Autodesk Inventor part; units mm, degrees
ref_plane "YZ Plane" through (0, 0, 0) normal (1, 0, 0) x (0, 1, 0)
ref_plane "XZ Plane" through (0, 0, 0) normal (0, 1, 0) x (-1, 0, 0)
ref_plane "XY Plane" through (0, 0, 0) normal (0, 0, 1) x (1, 0, 0)
sketch "Sketch1" plane through (0, 0, 0) normal (0, 0, 1) x (1, 0, 0)
  circle A0 centre (0, 0) radius 6.35
  dimension "d0" = 12.7
extrude "Extrusion1" add sketch "Sketch1" along normal blind 9.652
sketch "Sketch2" plane through (0, 0, 0) normal (0, 0, -1) x (-1, 0, 0)
  circle A0 centre (0, 0) radius 3.302
  dimension "d3" = 6.604
extrude "Extrusion2" add sketch "Sketch2" along normal blind 3.048
chamfer "Chamfer1" distance 0.762 angle 45 1 edges at (-6.35, 0, 9.652) measured on face at (-1.8127, -0.4771, 9.652)
sketch "Sketch3" plane through (0, 0, 9.652) normal (0, 0, 1) x (1, 0, 0)
  circle A0 centre (0, 0) radius 6.35
  line L0 (3.175, 5.4993) -> (6.35, 0)
  line L1 (6.35, 0) -> (3.175, -5.4993)
  line L2 (3.175, -5.4993) -> (-3.175, -5.4993)
  line L3 (-3.175, -5.4993) -> (-6.35, 0)
  line L4 (-6.35, 0) -> (-3.175, 5.4993)
  line L5 (-3.175, 5.4993) -> (3.175, 5.4993)
  line L6 (-10.603, 0.0515) -> (9.8262, 0.0515) construction
extrude "Extrusion3" cut sketch "Sketch3" against normal up to surface (9.652 mm away) contours L0 A0 | A0 L1 | L5 A0 | A0 L2 | L4 A0 | A0 L3
sketch "Sketch5" plane through (0, 0, -3.048) normal (0, 0, -1) x (-1, 0, 0)
  circle A0 centre (0, 0) radius 3.937
  dimension "d15" = 7.874
extrude "Extrusion5" [suppressed]
chamfer "Chamfer2" [suppressed]
thread "Thread1"
sketch "Sketch6" plane through (-3.175, 5.4993, 11.0682) normal (0, 1, 0) x (1, 0, 0)
  line L0 (0, 0) -> (0, 9.652)
  line L1 (0, 7.7662) -> (6.35, 7.7662)
  line L2 (6.35, 0) -> (6.35, 9.652)
  line L3 (-0.762, 14.1162) -> (7.112, 14.1162)
  line L4 (-0.762, 14.1162) -> (7.112, 14.1162)
  point P0 (3.175, 0)
  point P1 (3.175, 7.7662)
  dimension "d25" = 6.35
  dimension "d36" = 6.35
  dimension "d37" = 3.175
  dimension "d45" = 0
hole "Hole1" [suppressed]
pattern_circular "Circular Pattern1" [suppressed]
sketch "Sketch7" plane through (0, 0, 9.652) normal (0, 0, 1) x (1, 0, 0)
  point P0 (0, 0)
  point P1 (0, 0)
hole "Hole2" [suppressed]
properties part number "13_5_CylinderBase"
Build history of the part. All positions in model axes, mm. A direction names the side the tool comes from. Round coordinates to 2 decimals unless told otherwise and drop trailing zeros. Loops run counter-clockwise (first coordinate to the right, second up) from the corner with the lowest first, then second, coordinate; pieces in that order, holes last. Notation, with made-up numbers: (66, 4.5) -> (97, 4.5) arc R31 cw to (97, 28.5) -> close; hole circle Ø11 at (33.25, 73). An arc over 180 degrees is marked (long way). Answer in a Markdown table with one row per item.
Item 1: Drill centre lines: L1, parallel to Z at x = -1, y = -4.25; L2, parallel to X at y = -4, z = 6; L3, parallel to X at y = 3.25, z = 2.5. Where is each one in solid material? Low to high. Write a range as [from, to].
Answers below:
| item | result |
|---|---|
| L1 | z = [0, 9.65] |
| L2 | x = [-4.04, 4.04] |
| L3 | x = [-4.47, 4.47] |
Item 2: Which spindle directions (+Z, -Z, +X, -X, +Y, -Y) get a long thin tool onto all of the face, cutting with end or side? Do faces 1 (the flat face through (3, 3, 0)), 2 (the flat face through (4.74, 2.79, 4.89)). Say none if no direction does.
Answers below:
| item | result |
|---|---|
| face 1 | -Z |
| face 2 | +Z, -Z, +X, +Y |
Item 3: Saw through at A-A (x = 0). Write the cut outline in (y, z), and give its area (3 significant figures).
Answers below:
| item | result |
|---|---|
| outline | (-5.5, 0) -> (-3.3, 0) -> (-3.3, -3.05) -> (3.3, -3.05) -> (3.3, 0) -> (5.5, 0) -> (5.5, 9.65) -> (-5.5, 9.65) -> close |
| area | 126 mm² |
Item 4: Saw through at C-C (z = 5.75). Write the cut outline in (x, y) (3 decimals).
Answers below:
| item | result |
|---|---|
| outline | (-6.35, 0) -> (-3.175, -5.499) -> (3.175, -5.499) -> (6.35, 0) -> (3.175, 5.499) -> (-3.175, 5.499) -> close |
Item 5: Saw through at B-B (y = 2.5). Write the cut outline in (x, z).
Answers below:
| item | result |
|---|---|
| outline | (-4.91, 0) -> (-2.16, 0) -> (-2.16, -3.05) -> (2.16, -3.05) -> (2.16, 0) -> (4.91, 0) -> (4.91, 9.65) -> (-4.91, 9.65) -> close |
Item 6: Saw through at D-D (z = -1.5). Write the cut outline in (x, y), and give its area (3 significant figures).
Answers below:
| item | result |
|---|---|
| outline | circle Ø6.6 at (0, 0) |
| area | 34.3 mm² |
Item 7: Pin check, flat tip, straight feed: pin 1 (4 mm diameter, centred on y = 0.5, z = 4, fed in from +X). Stop position of the tip, or through.
Answers below:
| item | result |
|---|---|
| pin 1 | stops at x = 6.35 |
